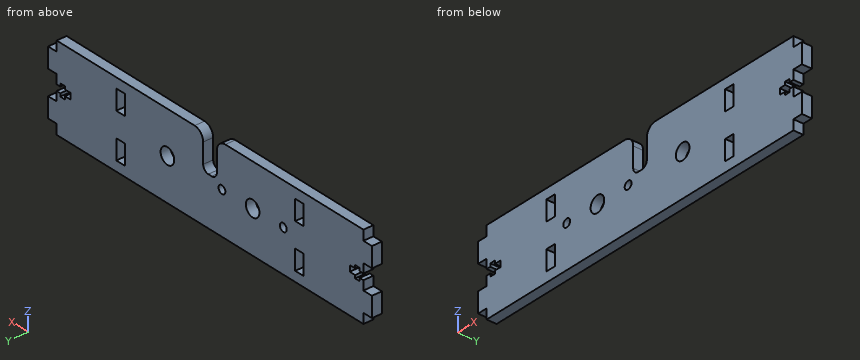
from build123d import *

# Parameters (mm, degrees)
SKETCH_1_R      = 4
SKETCH_1_R_2    = 2
SKETCH_1_W      = 5
SKETCH_1_H      = 10
EXTRUDE_1_DEPTH = 5


with BuildPart() as part:
    # 草图1 → 凸台-拉伸1 (new body)
    with BuildSketch(Plane(origin=(0, 0, 0), x_dir=(1, 0, 0), z_dir=(0, 1, 0))):
        with BuildLine():
            Line((-87.471894738, -35.047998618), (-6.471894738, -35.047998618))
            ThreePointArc((-6.471894738, -35.047998618), (-2.936360832, -33.583532524), (-1.471894738, -30.047998618))
            Line((-1.471894738, -30.047998618), (-1.471894738, -20.047998618))
            ThreePointArc((-1.471894738, -20.047998618), (-0.593215082, -17.926678275), (1.528105262, -17.047998618))
            Line((1.528105262, -17.047998618), (3.528105262, -17.047998618))
            ThreePointArc((3.528105262, -17.047998618), (5.649425606, -17.926678275), (6.528105262, -20.047998618))
            Line((6.528105262, -20.047998618), (6.528105262, -30.047998618))
            ThreePointArc((6.528105262, -30.047998618), (7.992571356, -33.583532524), (11.528105262, -35.047998618))
            Line((11.528105262, -35.047998618), (92.528105262, -35.047998618))
            Line((92.528105262, -35.047998618), (92.528105262, -30.047998618))
            Line((92.528105262, -30.047998618), (97.528105262, -30.047998618))
            Line((97.528105262, -30.047998618), (97.528105262, -20.047998618))
            Line((97.528105262, -20.047998618), (92.528105262, -20.047998618))
            Line((92.528105262, -20.047998618), (92.528105262, -15.388953653))
            Line((92.528105262, -15.388953653), (90.378105262, -15.388953653))
            Line((90.378105262, -15.388953653), (90.378105262, -16.897998618))
            Line((90.378105262, -16.897998618), (87.678105262, -16.897998618))
            Line((87.678105262, -16.897998618), (87.678105262, -15.388953653))
            Line((87.678105262, -15.388953653), (84.528105262, -15.388953653))
            Line((84.528105262, -15.388953653), (84.528105262, -12.397998618))
            Line((84.528105262, -12.397998618), (87.678105262, -12.397998618))
            Line((87.678105262, -12.397998618), (87.678105262, -10.897998618))
            Line((87.678105262, -10.897998618), (90.378105262, -10.897998618))
            Line((90.378105262, -10.897998618), (90.378105262, -12.397998618))
            Line((90.378105262, -12.397998618), (92.528105262, -12.397998618))
            Line((92.528105262, -12.397998618), (92.528105262, -7.747998618))
            Line((92.528105262, -7.747998618), (97.528105262, -7.747998618))
            Line((97.528105262, -7.747998618), (97.528105262, 2.252001382))
            Line((97.528105262, 2.252001382), (92.528105262, 2.252001382))
            Line((92.528105262, 2.252001382), (92.528105262, 7.252001382))
            Line((92.528105262, 7.252001382), (-87.471894738, 7.252001382))
            Line((-87.471894738, 7.252001382), (-87.471894738, 2.252001382))
            Line((-87.471894738, 2.252001382), (-92.471894738, 2.252001382))
            Line((-92.471894738, 2.252001382), (-92.471894738, -7.747998618))
            Line((-92.471894738, -7.747998618), (-87.471894738, -7.747998618))
            Line((-87.471894738, -7.747998618), (-87.471894738, -12.397998618))
            Line((-87.471894738, -12.397998618), (-85.321894738, -12.397998618))
            Line((-85.321894738, -12.397998618), (-85.321894738, -10.897998618))
            Line((-85.321894738, -10.897998618), (-82.621894738, -10.897998618))
            Line((-82.621894738, -10.897998618), (-82.621894738, -12.397998618))
            Line((-82.621894738, -12.397998618), (-79.471894738, -12.397998618))
            Line((-79.471894738, -12.397998618), (-79.471894738, -15.388953653))
            Line((-79.471894738, -15.388953653), (-82.621894738, -15.388953653))
            Line((-82.621894738, -15.388953653), (-82.621894738, -16.897998618))
            Line((-82.621894738, -16.897998618), (-85.321894738, -16.897998618))
            Line((-85.321894738, -16.897998618), (-85.321894738, -15.388953653))
            Line((-85.321894738, -15.388953653), (-87.471894738, -15.388953653))
            Line((-87.471894738, -15.388953653), (-87.471894738, -20.047998618))
            Line((-87.471894738, -20.047998618), (-92.471894738, -20.047998618))
            Line((-92.471894738, -20.047998618), (-92.471894738, -30.047998618))
            Line((-92.471894738, -30.047998618), (-87.471894738, -30.047998618))
            Line((-87.471894738, -30.047998618), (-87.471894738, -35.047998618))
        make_face()
        with Locations(Location((-22.471894738, -13.897998618, 0), (0, 0, 270))):
            Circle(SKETCH_1_R, mode=Mode.SUBTRACT)
        with Locations(Location((27.528105262, -13.897998618, 0), (0, 0, 270))):
            Circle(SKETCH_1_R, mode=Mode.SUBTRACT)
        with Locations(Location((-40.471894738, -13.897998618, 0), (0, 0, 270))):
            Circle(SKETCH_1_R_2, mode=Mode.SUBTRACT)
        with Locations(Location((-4.471894738, -13.897998618, 0), (0, 0, 270))):
            Circle(SKETCH_1_R_2, mode=Mode.SUBTRACT)
        with Locations((-49.971894738, -2.747998618)):
            Rectangle(SKETCH_1_W, SKETCH_1_H, mode=Mode.SUBTRACT)
        with Locations((-49.971894738, -25.047998618)):
            Rectangle(SKETCH_1_W, SKETCH_1_H, mode=Mode.SUBTRACT)
        with Locations((55.028105262, -25.047998618)):
            Rectangle(SKETCH_1_W, SKETCH_1_H, mode=Mode.SUBTRACT)
        with Locations((55.028105262, -2.747998618)):
            Rectangle(SKETCH_1_W, SKETCH_1_H, mode=Mode.SUBTRACT)
    extrude(amount=EXTRUDE_1_DEPTH)


solid = part.part
Part model, mm, in its own coordinate system. Round coordinates to 2 decimals unless told otherwise and drop trailing zeros. Order: outer loops, then holes, each group sorted by start corner. A loop starts at its lowest first (then second) coordinate and runs counter-clockwise, first axis right, second up. Notation, with made-up numbers: (27, 69) -> (48, 69) arc R18 ccw to (48, 75) -> close; hole circle Ø1 at (-14, -22.5). An arc over 180 degrees is marked (long way). Put each result on its own line as item: value.
Q1. Band-saw the part on B-B (z = 4.5). Give the cut face in (x, y), and give its area (3 significant figures).
From the geometry:
outline: (-92.47, 0) -> (-52.47, 0) -> (-52.47, 5) -> (-92.47, 5) -> close; (-47.47, 0) -> (52.53, 0) -> (52.53, 5) -> (-47.47, 5) -> close; (57.53, 0) -> (97.53, 0) -> (97.53, 5) -> (57.53, 5) -> close
area: 900 mm2
Q2. Pin check, flat tips, straight feed: pin 1 Ø1.5 at (x, y) = (95.5, 2.5) entering from -Z; pin 2 Ø10 at (x, z) = (4.5, 27.5) entering from +Y; pin 3 Ø0.5 at (y, z) = (3.5, 16.5) entering from -X; pin 4 Ø1.5 at (y, z) = (1, 10) entering from +X. Stop position of each tip, or through.
From the geometry:
pin 1: stops at z = -2.25
pin 2: stops at y = 5
pin 3: stops at x = -87.47
pin 4: stops at x = 92.53
Q3. Band-saw the part on C-C (y = 2.85). State how many separate pieces and enclosed holes the cut face has, and give its area (3 significant figures).
From the geometry:
separate pieces: 1
enclosed holes: 8
area: 7,270 mm2
Q4. Band-saw the part on A-A (z = 26.5). Give the cut face in (x, y), and give its area (3 significant figures).
From the geometry:
outline: (-92.47, 0) -> (-52.47, 0) -> (-52.47, 5) -> (-92.47, 5) -> close; (-47.47, 0) -> (-1.47, 0) -> (-1.47, 5) -> (-47.47, 5) -> close; (6.53, 0) -> (52.53, 0) -> (52.53, 5) -> (6.53, 5) -> close; (57.53, 0) -> (97.53, 0) -> (97.53, 5) -> (57.53, 5) -> close
area: 860 mm2
Q5. Wall check: line 1 (X direction, y = 1.65, z = 20.5); line 2 (X direction, y = 1.9, z = 6.5); line 3 (X direction, y = 4.1, z = 13). Give the ranges that are in metal, low to high. Write a range as [from, to].
From the geometry:
line 1: x = [-92.47, -52.47], [-47.47, -1.47], [6.53, 52.53], [57.53, 97.53]
line 2: x = [-92.47, -52.47], [-47.47, 52.53], [57.53, 97.53]
line 3: x = [-79.47, -42.26], [-38.68, -26.37], [-18.57, -6.26], [-2.68, 23.63], [31.43, 84.53]
